Can you work these out from the model? Positions are in its coordinate system, mm. Face numbers are marked on the shaded views. A direction names the side the tool comes from. Round coordinates to 2 decimals unless told otherwise and drop trailing zeros. Order: outer loops, then holes, each group sorted by start corner. A loop starts at its lowest first (then second) coordinate and runs counter-clockwise, first axis right, second up.
Q1. If we section it at D-D (x = -2): Please give me the cut outline in (y, z).
Q2. If I drill on line 1 (Z direction, x = 0, y = 1.85); line 2 (Y direction, x = -1.75, z = -2.5); line 3 (Y direction, x = 1, z = -4.5), over which ranges is the centre line in solid material (lowest first)?
Q3. If we section it at C-C (y = 7.25): Please give me the cut outline in (x, z), plus the area to 3 significant figures.
Q4. We'd pull the mould along Z, two halves only. Please class the marked faces 4, 5 and 6: pulls with the +Z half, pulls with the -Z half, needs draft (parallel to the pull), parting line crosses it, or undercut.
Q5. If we section it at A-A (x = 0): Please give me the cut outline in (y, z).
Q6. Will these pins go through, and if not, where does the flat tip stop? P1, Ø5, axis at x = -1, y = 15.5, coming from the -Z side; P2, Ø5.5, axis at x = 0, z = -1.5, coming from the -Y side; P3, Ø1, axis at y = 13, z = -3.5, coming from the +X side; P4, Ø3, axis at y = 8.5, z = -0.5, coming from the +X side.
Q7. For the marked faces 1, 2 and 3, which set-ups out of +Z, -Z, +X, -X, +Y, -Y let a thin tool reach every point of the face, with its end or its side?
Q8. If we section it at B-B (z = 0): Please give me the cut outline in (x, y).
from build123d import *

# Parameters (mm, degrees)
SKETCH_1_R          = 5
EXTRUDE_1_DEPTH     = 4
SKETCH_2_R          = 3.8
EXTRUDE_2_DEPTH     = 14
SKETCH_3_R          = 3.5
SKETCH_3_R_2        = 0.75
CUT_EXTRUDE_1_DEPTH = 3


with BuildPart() as part:
    # 草图1 → 凸台-拉伸1 (new body)
    with BuildSketch(Plane(origin=(0, 0, 0), x_dir=(1, 0, 0), z_dir=(0, 1, 0))):
        Circle(SKETCH_1_R)
    extrude(amount=EXTRUDE_1_DEPTH)

    # 草图2 → 凸台-拉伸2 (add)
    with BuildSketch(Plane(origin=(0, 4, 0), x_dir=(1, 0, 0), z_dir=(0, 1, 0))):
        Circle(SKETCH_2_R)
    extrude(amount=EXTRUDE_2_DEPTH)

    # 草图3 → 切除-拉伸1 (cut)
    with BuildSketch(Plane.XZ):
        Circle(SKETCH_3_R)
        Circle(SKETCH_3_R_2, mode=Mode.SUBTRACT)
    extrude(amount=-CUT_EXTRUDE_1_DEPTH, mode=Mode.SUBTRACT)


solid = part.part
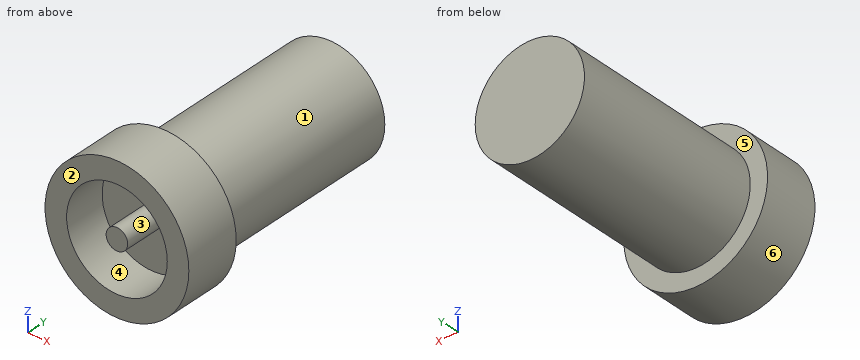
Solution:
1. outline: (0, -4.58) - (4, -4.58) - (4, -3.23) - (18, -3.23) - (18, 3.23) - (4, 3.23) - (4, 4.58) - (0, 4.58) - (0, 2.87) - (3, 2.87) - (3, -2.87) - (0, -2.87) - close
2. line 1: z = -5 to -3.5, -0.75 to 0.75, 3.5 to 5
2. line 2: y = 3 to 18
2. line 3: y = 0 to 4
3. outline: circle Ø7.6 at (0, 0)
3. area: 45.4 mm2
4. face 4: undercut
4. face 5: needs draft
4. face 6: parting line crosses it
5. outline: (0, -5) - (4, -5) - (4, -3.8) - (18, -3.8) - (18, 3.8) - (4, 3.8) - (4, 5) - (0, 5) - (0, 3.5) - (3, 3.5) - (3, 0.75) - (0, 0.75) - (0, -0.75) - (3, -0.75) - (3, -3.5) - (0, -3.5) - close
6. P1: stops at z = -3.8
6. P2: stops at y = 0
6. P3: stops at x = 2.33
6. P4: stops at x = 3.8
7. face 1: +Y
7. face 2: +Z, -Z, +X, -X, -Y
7. face 3: -Y
8. outline: (-5, 0) - (-3.5, 0) - (-3.5, 3) - (-0.75, 3) - (-0.75, 0) - (0.75, 0) - (0.75, 3) - (3.5, 3) - (3.5, 0) - (5, 0) - (5, 4) - (3.8, 4) - (3.8, 18) - (-3.8, 18) - (-3.8, 4) - (-5, 4) - close
